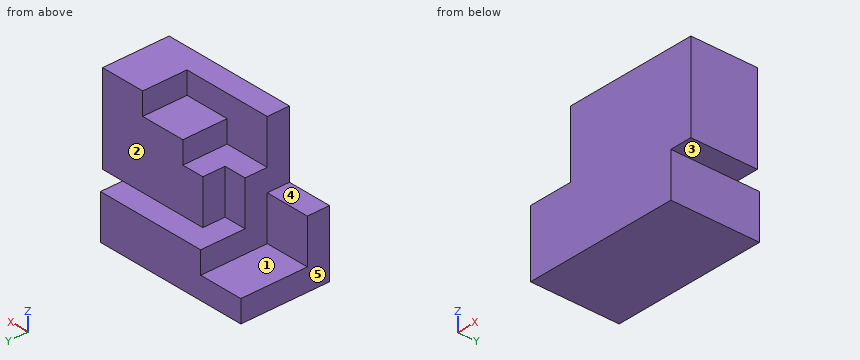
```python
from build123d import *

# Parameters (mm, degrees)
BOSS_EXTRUDE1_DEPTH = 10
BOSS_EXTRUDE2_DEPTH = 20
BOSS_EXTRUDE3_DEPTH = 10
SKETCH4_W           = 10
SKETCH4_H           = 26.291217747
CUT_EXTRUDE1_DEPTH  = 10


with BuildPart() as part:
    # Sketch1 → Boss-Extrude1 (new body)
    with BuildSketch(Plane(origin=(0, 0, 0), x_dir=(1, 0, 0), z_dir=(0, 1, 0))):
        Polygon((0, 0), (-10, 0), (-10, 20), (-80, 20), (-80, -10), (-60, -10), (-60, -40), (0, -40), align=None)
    extrude(amount=BOSS_EXTRUDE1_DEPTH)

    # Sketch2 → Boss-Extrude2 (add)
    with BuildSketch(Plane(origin=(0, 10, 0), x_dir=(1, 0, 0), z_dir=(0, 1, 0))):
        Polygon((-10, 20), (-10, 0), (0, 0), (0, -40), (-20, -40), (-20, -30), (-40, -30), (-40, -20), (-60, -20), (-60, -10), (-60, 10), (-80, 10), (-80, 20), (-60, 20), align=None)
    extrude(amount=BOSS_EXTRUDE2_DEPTH)

    # Sketch3 → Boss-Extrude3 (add)
    with BuildSketch(Plane(origin=(0, 30, 0), x_dir=(1, 0, 0), z_dir=(0, 1, 0))):
        Polygon((-80, 20), (-10, 20), (-10, 0), (-60, 0), (-60, 10), (-80, 10), align=None)
    extrude(amount=BOSS_EXTRUDE3_DEPTH)

    # Sketch4 → Cut-Extrude1 (cut)
    with BuildSketch(Plane(origin=(0, 30, 0), x_dir=(1, 0, 0), z_dir=(0, 1, 0))):
        with Locations((-55, -13.145608874)):
            Rectangle(SKETCH4_W, SKETCH4_H)
    extrude(amount=-CUT_EXTRUDE1_DEPTH, mode=Mode.SUBTRACT)


solid = part.part
```
Can you work these out from the model? Positions are in its coordinate system, mm. Face numbers are marked on the shaded views. A direction names the side the tool comes from. Coordinates: 2 decimals unless noted, no trailing zeros. Loops run counter-clockwise (first coordinate to the right, second up) from the corner with the lowest first, then second, coordinate; pieces in that order, holes last. Notation, with made-up numbers: (-18, 72.25) -> (-3, 72.25) arc R28 cw to (-3, 90.25) -> close; hole circle Ø7 at (-1.5, -1.5). An arc over 180 degrees is marked (long way). Put each result on its own line as item: value. Start each with the question number.
Q1. I want a section at D-D (z = 33.5). Write out the boundary of the cut face in (x, y).
Q2. If I drill on line 1 (Y direction, x = -41.5, z = 3.5); line 2 (Z direction, x = -24.5, y = 12); line 3 (Y direction, x = -44, z = 21), over which ranges is the centre line in solid material (lowest first)? Write a range as [from, to].
Q3. I want a section at B-B (y = 27). Write out the boundary of the cut face in (x, z), plus the area to 3 significant figures.
Q4. I want a section at C-C (x = -39). Write out the boundary of the cut face in (y, z).
Q5. I'm going to push flat-ended pins straight in: P1, Ø22, axis at x = -68, z = 0.5, coming from the +Y side; P2, Ø5, axis at x = -69, z = 13, coming from the +Y side; P3, Ø10, axis at y = 15.5, z = -14, coming from the +X side; P4, Ø5, axis at y = 25.5, z = 1.5, coming from the -X side. Where does each tip first touch, or does it pass through?
Q6. I want a section at A-A (z = 6). Write out the boundary of the cut face in (x, y), plus the area to 3 significant figures.
Q7. For the marked faces 1, 2, 3, 4 and 5, which set-ups out of +Z, -Z, +X, -X, +Y, -Y let a thin tool reach every point of the face, with its end or its side?
Taken from the geometry:
1. outline: (-60, 0) -> (0, 0) -> (0, 30) -> (-20, 30) -> (-20, 10) -> (-60, 10) -> close
2. line 1: y = [0, 30]
2. line 2: z = [-20, 30]
2. line 3: y = [0, 10]
3. outline: (-80, -20) -> (-10, -20) -> (-10, 0) -> (0, 0) -> (0, 40) -> (-20, 40) -> (-20, 30) -> (-40, 30) -> (-40, 20) -> (-50, 20) -> (-50, 0) -> (-60, 0) -> (-60, -10) -> (-80, -10) -> close
3. area: 2,800 mm2
4. outline: (0, -20) -> (40, -20) -> (40, 0) -> (30, 0) -> (30, 30) -> (10, 30) -> (10, 40) -> (0, 40) -> close
5. P1: stops at y = 40
5. P2: passes through
5. P3: stops at x = -10
5. P4: stops at x = -60
6. outline: (-80, 0) -> (0, 0) -> (0, 30) -> (-50, 30) -> (-50, 20) -> (-60, 20) -> (-60, 10) -> (-80, 10) -> close
6. area: 1,900 mm2
7. face 1: +Z, -X, +Y
7. face 2: +Z, +X, -X, +Y
7. face 3: -Z, +X, +Y, -Y
7. face 4: +Z, -X, +Y, -Y
7. face 5: +Z, -Z, -X, +Y, -Y
